from build123d import *

# Parameters (mm, degrees)
SKETCH2_W                    = 82.24
SKETCH2_H                    = 42.26
BOSS_EXTRUDE1_DEPTH          = 60
FILLET1_R                    = 3
SKETCH5_OUTSIDE_W            = 106.284
SKETCH5_OUTSIDE_H            = 66.304
CUT_EXTRUDE2_DEPTH           = 40
CUT_EXTRUDE3_DEPTH           = 76.745173444
FILLET2_R                    = 3
FILLET3_R                    = 3
M10_TAPPED_HOLE1_D           = 8.5
M10_TAPPED_HOLE1_DEPTH       = 16.946342369
M10_TAPPED_HOLE1_CSINK_D     = 10.05
M10_TAPPED_HOLE1_CSINK_ANGLE = 90
M10_TAPPED_HOLE1_TIP         = 2.553657631


with BuildPart() as part:
    # Sketch2 → Boss-Extrude1 (new body)
    with BuildSketch(Plane(origin=(0, 0, 0), x_dir=(1, 0, 0), z_dir=(0, 1, 0))):
        Rectangle(SKETCH2_W, SKETCH2_H)
    extrude(amount=-BOSS_EXTRUDE1_DEPTH)

    # Fillet1
    fillet1_edges = [part.edges().sort_by_distance(p)[0] for p in [
        (41.12, -30, 21.13),
        (-41.12, -30, 21.13),
        (-41.12, -30, -21.13),
        (41.12, -30, -21.13),
    ]]
    fillet(fillet1_edges, radius=FILLET1_R)

    # Sketch5 outside → Cut-Extrude2 (cut)
    with BuildSketch(Plane.XZ.offset(60)):
        Rectangle(SKETCH5_OUTSIDE_W, SKETCH5_OUTSIDE_H)
        with BuildLine():
            Line((19, -21.13), (30.13, -21.13))
            Line((30.13, -21.13), (30.13, 21.13))
            Line((30.13, 21.13), (-41.12, 21.13))
            Line((-41.12, 21.13), (-41.12, -21.13))
            Line((-41.12, -21.13), (-19, -21.13))
            Line((-19, -21.13), (-19, -15))
            ThreePointArc((-19, -15), (-17.242640687, -10.757359313), (-13, -9))
            Line((-13, -9), (-9, -9))
            ThreePointArc((-9, -9), (-6.878679656, -8.121320344), (-6, -6))
            Line((-6, -6), (-6, 10.13))
            ThreePointArc((-6, 10.13), (0, 16.13), (6, 10.13))
            Line((6, 10.13), (6, -6))
            ThreePointArc((6, -6), (6.878679656, -8.121320344), (9, -9))
            Line((9, -9), (13, -9))
            ThreePointArc((13, -9), (17.242640687, -10.757359313), (19, -15))
            Line((19, -15), (19, -21.13))
        make_face(mode=Mode.SUBTRACT)
    extrude(amount=-CUT_EXTRUDE2_DEPTH, mode=Mode.SUBTRACT)

    # Sketch6 → Cut-Extrude3 (cut, through all)
    with BuildSketch(Plane.XZ.offset(60)):
        with BuildLine():
            Line((-13, -9), (-9, -9))
            ThreePointArc((-9, -9), (-6.878679656, -8.121320344), (-6, -6))
            Line((-6, -6), (-6, 10.13))
            ThreePointArc((-6, 10.13), (0, 16.13), (6, 10.13))
            Line((6, 10.13), (6, -6))
            ThreePointArc((6, -6), (6.878679656, -8.121320344), (9, -9))
            Line((9, -9), (13, -9))
            ThreePointArc((13, -9), (17.242640687, -10.757359313), (19, -15))
            Line((19, -15), (19, -21.13))
            Line((19, -21.13), (-19, -21.13))
            Line((-19, -21.13), (-19, -15))
            ThreePointArc((-19, -15), (-17.242640687, -10.757359313), (-13, -9))
        make_face()
    extrude(amount=-CUT_EXTRUDE3_DEPTH, mode=Mode.SUBTRACT)

    # Fillet2
    fillet2_edges = [part.edges().sort_by_distance(p)[0] for p in [
        (30.13, -40, 21.13),
        (30.13, -40, -21.13),
    ]]
    fillet(fillet2_edges, radius=FILLET2_R)

    # Fillet3
    # the kernel refuses this fillet: 3 mm, written as the material it adds along each edge
    with BuildSketch(Plane(origin=(30.13, -20, -18.13), x_dir=(0, -1, 0), z_dir=(0, 0, 1))) as fillet3_piece_1:
        with BuildLine():
            CenterArc((FILLET3_R, FILLET3_R), FILLET3_R, 180, 90)
            Line((0, FILLET3_R), (0, 0))
            Line((0, 0), (FILLET3_R, 0))
        make_face()
    extrude(amount=36.26)
    with BuildSketch(Plane(origin=(27.13, -20, 18.13), x_dir=(-0.5976672776328266, 0, -0.801744239297649), z_dir=(0.801744239297649, 0, -0.5976672776328266))) as fillet3_piece_2_section:
        with BuildLine():
            CenterArc((3 + FILLET3_R, -FILLET3_R), FILLET3_R, 90, 90)
            Line((3, -FILLET3_R), (3, 0))
            Line((3, 0), (3 + FILLET3_R, 0))
        make_face()
    fillet3_piece_2 = revolve(axis=Axis((27.13, -20, 18.13), (0, 1, 0)), revolution_arc=233.296989237, mode=Mode.PRIVATE)
    fillet3_piece_2 = split(fillet3_piece_2, bisect_by=Plane(origin=(29.379816868, -20.934884818, 21.13), z_dir=(0, 0, -1)), keep=Keep.TOP, mode=Mode.PRIVATE)
    add(fillet3_piece_2)
    with BuildSketch(Plane(origin=(27.13, -20, -18.13), x_dir=(-0.5976672776328287, 0, 0.8017442392976475), z_dir=(0.8017442392976475, 0, 0.5976672776328287))) as fillet3_piece_3_section:
        with BuildLine():
            CenterArc((3 + FILLET3_R, FILLET3_R), FILLET3_R, 180, 90)
            Line((3 + FILLET3_R, 0), (3, 0))
            Line((3, 0), (3, FILLET3_R))
        make_face()
    fillet3_piece_3 = revolve(axis=Axis((27.13, -20, -18.13), (0, -1, 0)), revolution_arc=233.296989237, mode=Mode.PRIVATE)
    fillet3_piece_3 = split(fillet3_piece_3, bisect_by=Plane(origin=(29.379816762, -20.934885263, -21.13), z_dir=(0, 0, 1)), keep=Keep.TOP, mode=Mode.PRIVATE)
    add(fillet3_piece_3)

    # M10 Tapped Hole1
    with Locations(Plane(origin=(0, 0, 0), x_dir=(1, 0, 0), z_dir=(0, 1, 0))):
        with Locations((28.62, 0), (-28.62, 0)):
            CounterSinkHole(M10_TAPPED_HOLE1_D / 2, M10_TAPPED_HOLE1_CSINK_D / 2, depth=M10_TAPPED_HOLE1_DEPTH, counter_sink_angle=M10_TAPPED_HOLE1_CSINK_ANGLE)
            with Locations((0, 0, -(M10_TAPPED_HOLE1_DEPTH + M10_TAPPED_HOLE1_TIP / 2))):  # 118° drill point
                Cone(0, M10_TAPPED_HOLE1_D / 2, M10_TAPPED_HOLE1_TIP, mode=Mode.SUBTRACT)


solid = part.part
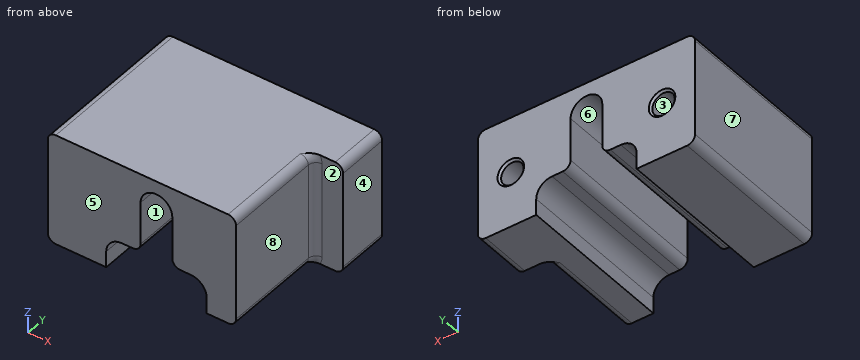
The model under review builds one solid part; all positions refer to its coordinate system, in mm. Face numbers are marked on the shaded views. A direction names the side the tool comes from. Coordinates: 2 decimals unless noted, no trailing zeros. Loops run counter-clockwise (first coordinate to the right, second up) from the corner with the lowest first, then second, coordinate; pieces in that order, holes last. Notation, with made-up numbers: M -33,61.25 L 1,61.25 A13 ccw 1,79.25 Z; hole C 83,-28 d8. An arc over 180 degrees is marked long. Put each result on its own line as item: value. Start each with the question number.
Q1. Add section D-D (y = -22). Write out the cut boundary in (x, z), and give its area (3 significant figures).
Q2. Add section A-A (y = -15). Write out the cut boundary in (x, z).
Q3. Wall thickness on line 1 (X direction, y = -41.5, z = -2); line 2 (Z direction, x = -28.62, y = -13.5); line 3 (Y direction, x = 36, z = -3): over which ranges is each line inside the solid? List them lowest first.
Q4. For the marked faces 1, 2, 3 and 4, list the 3-axis set-ups (+Z, -Z, +X, -X, +Y, -Y) from which the entire face can be reached by the end or side of a thin tool; tool diameter is ignored.
Q5. The part is to be moulded in two halves that separate along X. For the marked faces 5, 6, 7 and 8, say which applies: +X half, -X half, draft (parallel to the pull), parting line (faces both ways), or undercut.
Q6. Clearance check with flat-ended pins moving along their axes: pin 1 (4.5 mm diameter, centred on x = 35, z = -9, fed in from -Y); pin 2 (2 mm diameter, centred on y = -36.5, z = -3, fed in from +X); pin 3 (2 mm diameter, centred on x = -11.5, y = -30, fed in from -Z). State where each tip first meets the part, or that it passes through.
Q7. Add section B-B (y = -42). Write out the cut boundary in (x, z), and give its area (3 significant figures).
Q8. Add section C-C (x = 0). Write out the cut boundary in (y, z).
Answers:
1. outline: M -41.12,-18.13 A3 ccw -38.12,-21.13 L -19,-21.13 L -19,-15 A6 cw -13,-9 L -9,-9 A3 ccw -6,-6 L -6,10.13 A6 cw 6,10.13 L 6,-6 A3 ccw 9,-9 L 13,-9 A6 cw 19,-15 L 19,-21.13 L 28.16,-21.13 A3.17 ccw 30.3,-18.13 L 30.3,18.13 A3.17 ccw 28.16,21.13 L -38.12,21.13 A3 ccw -41.12,18.13 Z
1. area: 2,280 mm^2
2. outline: M -41.12,-18.13 A3 ccw -38.12,-21.13 L -19,-21.13 L -19,-15 A6 cw -13,-9 L -9,-9 A3 ccw -6,-6 L -6,10.13 A6 cw 6,10.13 L 6,-6 A3 ccw 9,-9 L 13,-9 A6 cw 19,-15 L 19,-21.13 L 38.12,-21.13 A3 ccw 41.12,-18.13 L 41.12,18.13 A3 ccw 38.12,21.13 L -38.12,21.13 A3 ccw -41.12,18.13 Z; hole C -28.62,0 d8.5; hole C 28.62,0 d8.5
3. line 1: x = -41.12 to -6, 6 to 30.13
3. line 2: z = -21.13 to -4.25, 4.25 to 21.13
3. line 3: y = -20 to 0
4. face 1: -Z, +Y, -Y
4. face 2: +Z, -Z, +X, -Y
4. face 3: +Y
4. face 4: +Z, -Z, +X, +Y, -Y
5. face 5: draft
5. face 6: undercut
5. face 7: -X half
5. face 8: +X half
6. pin 1: stops at y = -20.02
6. pin 2: stops at x = 30.13
6. pin 3: stops at z = -9
7. outline: M -41.12,-18.13 A3 ccw -38.12,-21.13 L -19,-21.13 L -19,-15 A6 cw -13,-9 L -9,-9 A3 ccw -6,-6 L -6,10.13 A6 cw 6,10.13 L 6,-6 A3 ccw 9,-9 L 13,-9 A6 cw 19,-15 L 19,-21.13 L 27.13,-21.13 A3 ccw 30.13,-18.13 L 30.13,18.13 A3 ccw 27.13,21.13 L -38.12,21.13 A3 ccw -41.12,18.13 Z
7. area: 2,270 mm^2
8. outline: M -60,16.13 L 0,16.13 L 0,21.13 L -60,21.13 Z
